Input: part model. Units: mm. Frame: model coordinates. Face numbers are marked on the shaded views. A direction names the side the tool comes from. Coordinates: 2 decimals unless noted, no trailing zeros. Write each loop counter-clockwise with the first axis right and the second up, starting at its lowest first coordinate (ties: lowest second). Pieces come first, ordered by that corner, then holes. Notation, with made-up numbers: (-40, -6.5) - (-25, -6.5) arc R13 cw to (-25, 3.5) - close; hole circle Ø11 at (3, 48). An arc over 180 degrees is marked (long way). Use a Markdown table: item, result. Add a question column.
Q1. Mould query, pull axis X, two halves, no side actions, for the marked faces 6, 7 and 8. Classes: released by +X, released by -X, zero draft, split by the parting line, or undercut.
Q2. Section query A-A (z = 32.5). Return the cut outline in (x, y), then the cut area to 3 significant figures.
Q3. Set-up query: the marked faces 1, 2, 3, 4 and 5. Return all of +Z, -Z, +X, -X, +Y, -Y with unobstructed straight access to the full face (end or side cutting, diameter ignored); none if empty.
Q4. Section query B-B (x = 25.4). Return the cut outline in (y, z), then the cut area to 3 significant figures.
Q5. Material intervals for probe 1 along X at (y, z) = (-16.5, 28.5); probe 2 along Z at (x, y) = (25.4, -25); probe 3 along X at (y, z) = (-6.75, 12), sorted ascending. Write a range as from..to.
Q6. Pin query (flat end, axial travel): P1, Ø4, axis at x = 19.5, y = -6, coming from the +Z side; P2, Ø0.6, axis at x = 18.5, y = -25, coming from the -Z side; P3, Ø1.8, axis at x = 9.5, y = -15.5, coming from the +Z side; P4, Ø7.5, axis at x = 25, z = 25, coming from the -Y side. Return the tip coordinate at first contact, or that it passes through.
Q7. Section query D-D (x = 13). Return the cut outline in (y, z) (3 decimals), then the cut area to 3 significant figures.
Q8. Section query C-C (x = 42). Return the cut outline in (y, z).
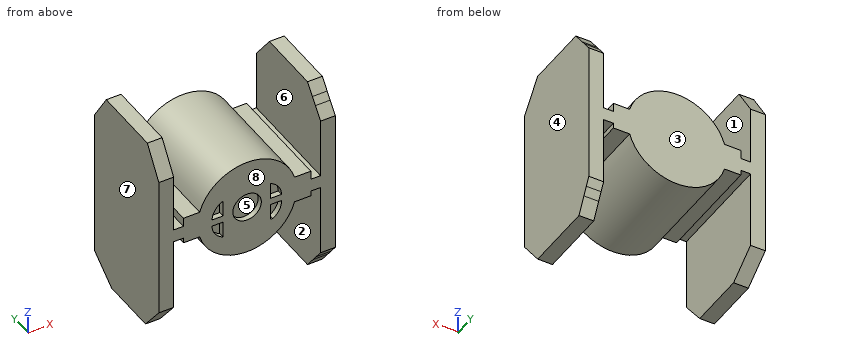
from build123d import *

# Parameters (mm, degrees)
F0_W     = 2.286
F0_H     = 3.048
F1_DEPTH = 25.4
F3_DEPTH = 12.7
F5_DEPTH = 12.7
F6_R     = 3.335139
F7_DEPTH = 1.27


with BuildPart() as f1:
    # F0 (on Front) → F1 (new body)
    with BuildSketch(Plane.XZ):
        Polygon((42.583782, 23.443561), (42.583782, 0), (46.038182, 0), (46.038182, 47.156759), (42.583782, 47.156759), (42.583782, 26.491561), align=None)
        Polygon((4.761818, 47.156759), (4.761818, 0), (8.216218, 0), (8.216218, 23.443561), (8.216218, 26.491561), (8.216218, 47.156759), align=None)
        with BuildLine():
            ThreePointArc((14.312218, 28.575), (13.86659, 25.4), (14.312218, 22.225))
            ThreePointArc((14.312218, 22.225), (25.4, 13.86659), (36.487782, 22.225))
            ThreePointArc((36.487782, 22.225), (36.82146, 23.79694), (36.93341, 25.4))
            ThreePointArc((36.93341, 25.4), (36.82146, 27.00306), (36.487782, 28.575))
            ThreePointArc((36.487782, 28.575), (25.4, 36.93341), (14.312218, 28.575))
        make_face()
        with Locations((9.359218, 24.967561)):
            Rectangle(F0_W, F0_H)
        with BuildLine():
            Line((10.502218, 26.491561), (10.502218, 23.443561))
            Line((10.502218, 23.443561), (10.502218, 22.225))
            Line((10.502218, 22.225), (14.312218, 22.225))
            ThreePointArc((14.312218, 22.225), (13.86659, 25.4), (14.312218, 28.575))
            Line((14.312218, 28.575), (10.502218, 28.575))
            Line((10.502218, 28.575), (10.502218, 26.491561))
        make_face()
        with BuildLine():
            Line((40.297782, 22.225), (40.297782, 23.443561))
            Line((40.297782, 23.443561), (40.297782, 26.491561))
            Line((40.297782, 26.491561), (40.297782, 28.575))
            Line((40.297782, 28.575), (36.487782, 28.575))
            ThreePointArc((36.487782, 28.575), (36.82146, 27.00306), (36.93341, 25.4))
            ThreePointArc((36.93341, 25.4), (36.82146, 23.79694), (36.487782, 22.225))
            Line((36.487782, 22.225), (40.297782, 22.225))
        make_face()
        with Locations((41.440782, 24.967561)):
            Rectangle(F0_W, F0_H)
    extrude(amount=F1_DEPTH)

    # F2 (on face) → F3 (cut)
    with BuildSketch(Plane.YZ.offset(46.038182)):
        Polygon((-25.4, 47.156759), (-25.4, 40.552066), (-23.363257, 43.158547), (-22.17105, 44.684251), (-20.238997, 47.156759), align=None)
        Polygon((0, 47.156759), (-5.161003, 47.156759), (-2.580502, 43.854412), (-1.72774, 42.763107), (0, 40.552066), align=None)
        Polygon((-1.957984, 3.705507), (-3.915968, 0), (0, 0), (0, 7.411013), (-0.994495, 5.528921), align=None)
        Polygon((-23.728574, 4.465718), (-25.4, 6.604693), (-25.4, 0), (-20.238997, 0), (-22.428798, 2.802356), align=None)
    extrude(amount=-F3_DEPTH, mode=Mode.SUBTRACT)

    # F4 (on face) → F5 (cut)
    with BuildSketch(Plane(origin=(4.761818, 0, 0), x_dir=(0, -1, 0), z_dir=(-1, 0, 0))):
        Polygon((0, 47.156759), (0, 40.144437), (4.59187, 47.156759), align=None)
        Polygon((25.4, 47.156759), (20.84787, 47.156759), (25.4, 40.118574), align=None)
        Polygon((25.4, 6.510113), (20.120194, 0), (25.4, 0), align=None)
        Polygon((6.716533, 0), (0, 5.01459), (0, 0), align=None)
    extrude(amount=-F5_DEPTH, mode=Mode.SUBTRACT)

    # F6 (on face) → F7 (cut)
    with BuildSketch(Plane.XZ.offset(25.4)):
        with Locations((25.4, 25.4)):
            Circle(F6_R)
        with BuildLine():
            ThreePointArc((19.747045, 29.21), (17.926817, 27.671819), (17.207045, 25.4))
            Line((17.207045, 25.4), (19.747045, 25.4))
            Line((19.747045, 25.4), (19.747045, 29.21))
        make_face()
        with BuildLine():
            Line((30.909679, 29.21), (30.909679, 25.4))
            Line((30.909679, 25.4), (33.449679, 25.4))
            ThreePointArc((33.449679, 25.4), (32.741123, 27.679296), (30.909679, 29.21))
        make_face()
        with BuildLine():
            Line((19.747045, 19.998197), (19.747045, 23.808197))
            Line((19.747045, 23.808197), (17.207045, 23.808197))
            ThreePointArc((17.207045, 23.808197), (17.898284, 21.517356), (19.747045, 19.998197))
        make_face()
        with BuildLine():
            Line((33.449679, 23.808197), (30.909679, 23.808197))
            Line((30.909679, 23.808197), (30.909679, 19.998197))
            Line((30.909679, 19.998197), (31.397671, 19.998197))
            ThreePointArc((31.397671, 19.998197), (32.955333, 21.616853), (33.449679, 23.808197))
        make_face()
    extrude(amount=-F7_DEPTH, mode=Mode.SUBTRACT)


solid = f1.part
Values follow:
| question | item | result |
|---|---|---|
| 1 | face 6 | undercut |
| 1 | face 7 | released by -X |
| 1 | face 8 | zero draft |
| 2 | outline | (4.76, -25.4) - (8.22, -25.4) - (8.22, 0) - (4.76, 0) - close; (16.31, -25.4) - (34.49, -25.4) - (34.49, 0) - (16.31, 0) - close; (42.58, -25.4) - (46.04, -25.4) - (46.04, 0) - (42.58, 0) - close |
| 2 | area | 637 mm2 |
| 3 | face 1 | +Z, +Y, -Y |
| 3 | face 2 | -Z, +Y, -Y |
| 3 | face 3 | +Z, -Z, +X, -X, +Y |
| 3 | face 4 | +Z, -Z, +X, +Y, -Y |
| 3 | face 5 | -Y |
| 4 | outline | (-25.4, 13.87) - (0, 13.87) - (0, 36.93) - (-25.4, 36.93) - (-25.4, 28.74) - (-24.13, 28.74) - (-24.13, 22.06) - (-25.4, 22.06) - close |
| 4 | area | 577 mm2 |
| 5 | probe 1 | 4.76..8.22, 10.5..40.3, 42.58..46.04 |
| 5 | probe 2 | 13.87..22.06, 28.74..36.93 |
| 5 | probe 3 | 4.76..8.22, 42.58..46.04 |
| 6 | P1 | z = 36.25 |
| 6 | P2 | z = 15.94 |
| 6 | P3 | z = 26.49 |
| 6 | P4 | y = -25.4 |
| 7 | outline | (-25.4, 22.225) - (0, 22.225) - (0, 28.575) - (-25.4, 28.575) - close |
| 7 | area | 161 mm2 |
| 8 | outline | (-25.4, 23.44) - (0, 23.44) - (0, 26.49) - (-25.4, 26.49) - close |
